from build123d import *

# Parameters (mm, degrees)
SKETCH1_W            = 2.6416
SKETCH1_H            = 4.6228
SKETCH1_W_2          = 9.525
SKETCH1_H_2          = 53.9369
SKETCH1_4_W          = 9.525
SKETCH1_4_H          = 53.9369
SKETCH1_4_W_2        = 2.6416
SKETCH1_4_H_2        = 4.6228
M6_TAPPED_HOLE1_D    = 5
M6_CLEARANCE_HOLE1_D = 6.6


with BuildPart() as part:
    # Sketch1 → Revolve1 (revolve)
    with BuildSketch(Plane(origin=(0, 0, 0), x_dir=(0, 0, -1), z_dir=(1, 0, 0)), mode=Mode.PRIVATE) as revolve1_sk:
        Polygon((0, 61.5696), (0, 79.375), (9.525, 79.375), (9.525, 60.2869), (13.97, 60.2869), (13.97, 57.5056), (19.05, 57.5056), (19.05, 60.2869), (23.495, 60.2869), (23.495, 57.5056), (28.575, 57.5056), (28.575, 60.2869), (38.1, 60.2869), (38.1, 53.9369), (9.525, 53.9369), (0, 53.9369), (0, 56.9468), (2.6416, 56.9468), (2.6416, 61.5696), align=None)
        with Locations((1.3208, 59.2582)):
            Rectangle(SKETCH1_W, SKETCH1_H)
        with Locations((4.7625, 26.96845)):
            Rectangle(SKETCH1_W_2, SKETCH1_H_2)
    revolve(revolve1_sk.sketch.rotate(Axis((0, 0, 0), (0, 0, -1)), 180), axis=Axis((0, 0, 0), (0, 0, -1)))

    # Sketch1<4> → Cut-Revolve1 (revolve, cut)
    with BuildSketch(Plane(origin=(0, 0, 0), x_dir=(0, 0, -1), z_dir=(1, 0, 0)), mode=Mode.PRIVATE) as cut_revolve1_sk:
        with Locations((4.7625, 26.96845)):
            Rectangle(SKETCH1_4_W, SKETCH1_4_H)
        with Locations((1.3208, 59.2582)):
            Rectangle(SKETCH1_4_W_2, SKETCH1_4_H_2)
    revolve(cut_revolve1_sk.sketch.rotate(Axis((0, 0, 0), (0, 0, -1)), 180), axis=Axis((0, 0, 0), (0, 0, -1)), mode=Mode.SUBTRACT)

    # M6 Tapped Hole1 (through all)
    with Locations(Plane.XY):
        with Locations((-60.491874454, 34.925), (0, 69.85), (60.491874454, 34.925), (60.491874454, -34.925), (0, -69.85), (-60.491874454, -34.925)):
            Hole(M6_TAPPED_HOLE1_D / 2)

    # M6 Clearance Hole1 (through all)
    with Locations(Plane.XY):
        with Locations((-69.85, 0), (0, 0), (-34.925, 60.491874454), (34.925, 60.491874454), (69.85, 0), (34.925, -60.491874454), (-34.925, -60.491874454)):
            Hole(M6_CLEARANCE_HOLE1_D / 2)


solid = part.part
Verification items for the finished model (mm, model axes). A direction names the side the tool comes from. Give positions to 0.01 mm unless a question says otherwise; leave off trailing zeros. Order: outer loops, then holes, each group sorted by start corner. A loop starts at its lowest first (then second) coordinate and runs counter-clockwise, first axis right, second up. Notation, with made-up numbers: M -15,70.25 L 34,70.25 A13 ccw 34,78.25 Z; hole C -11,-17.75 d2. An arc over 180 degrees is marked long. Use one line per item in the form item = value. Start each with the question number.
Q1. Section check A-A (x = -69.85). Enter the section's corners in (y, z) (3 decimals).
Q2. Section check C-C (x = 0). Count the separate pieces of the cut face and the enclosed holes in it, then the cut area to 3 significant figures.
Q3. Scan lines: line 1 along Z through (x, y) = (30.5, 49.5) (3 decimals); line 2 along Z through (x, y) = (71.5, 17.5) (3 decimals); line 3 along Y through (x, z) = (-44, -10). Record each from-to range of solid material in increasing order. Write a range as [from, to].
Q4. Section check B-B (z = -25.5). Enter the section's corners in (x, y).
Q5. Section check D-D (y = 69.85). Enter the section's corners in (x, z) (3 decimals).
Q6. Access from +Z, -Z, +X, -X, +Y, -Y to the whole of each face (thin tool, end or side, straight path). Record for faces 1 (the cylindrical face through (-17.27, -54.85, -16.55)), 2 (the cylindrical face through (-18.109, -57.503, -33.404)), 3 (the flat face through (50, -21, 0)).
Q7. Go/stop test with flat-tipped pins: pin 1 Ø8.5 at (x, y) = (34.92, 60.49) entering from +Z; pin 2 Ø8.5 at (x, y) = (-34.92, 60.49) entering from -Z (3 decimals); pin 3 Ø6 at (x, z) = (5, -15.5) entering from +Y; pin 4 Ø5 at (y, z) = (27, -30) entering from +X. Record where each tip stops, or that it passes through.
Q8. Mould release check, pull along Z, two halves, no side actions. Record for faces 4 (the flat face through (-53.3, -29, -9.525)), 5 (the flat face through (22, -53.3, -23.495)), 6 (the cylindrical face through (-18.109, -57.503, -21.304)), 7 (the flat face through (22, 53.3, -28.575)): +Z half, -Z half, draft (parallel to the pull), parting line (faces both ways), or undercut.
Evaluation:
q1.outline = M -37.701,-9.525 L -3.3,-9.525 L -3.3,0 L -37.701,0 Z; M 3.3,-9.525 L 37.701,-9.525 L 37.701,0 L 3.3,0 Z
q2.separate_pieces = 4
q2.enclosed_holes = 0
q2.area = 671 mm2
q3.line_1 = [-38.1, -28.575], [-23.495, -19.05], [-13.97, -2.642]
q3.line_2 = [-9.525, 0]
q3.line_3 = [-41.21, -31.2], [31.2, 41.21]
q4.outline = C 0,0 d115.01; hole C 0,0 d107.87
q5.outline = M -37.701,-9.525 L -2.5,-9.525 L -2.5,0 L -37.701,0 Z; M 2.5,-9.525 L 37.701,-9.525 L 37.701,0 L 2.5,0 Z
q6.face_1 = none
q6.face_2 = -Z
q6.face_3 = +Z, +X, -X, +Y, -Y
q7.pin_1 = 0
q7.pin_2 = -9.525
q7.pin_3 = 60.24
q7.pin_4 = 55.08
q8.face_4 = -Z half
q8.face_5 = undercut
q8.face_6 = draft
q8.face_7 = undercut
